Part model, mm, in its own coordinate system. A direction names the side the tool comes from. Round coordinates to 2 decimals unless told otherwise and drop trailing zeros. Loops run counter-clockwise (first coordinate to the right, second up) from the corner with the lowest first, then second, coordinate; pieces in that order, holes last.
1) Band-saw the part on C-C, the plane y = 65. Write the cut outline in (x, z).
2) Mould opens along Y. For faces 3 (the cylindrical face through (5.07, 55.357, -56.748)), 4 (the cylindrical face through (90.297, 5.07, -26.743)), 5 (the flat face through (115.07, 46.638, -102.915)) say: +Y half, -Y half, draft (parallel to the pull), parting line (faces both ways), or undercut.
3) Probe line 1 (X direction, y = 4.5, z = -20); line 2 (Z direction, x = 89.5, y = 9.5); line 3 (Y direction, x = 117, z = -60). List the from-to ranges inside material, lowest first.
4) Band-saw the part on B-B, the plane z = -20. Write the cut outline in (x, y).
5) Band-saw the part on D-D, the plane y = 52.5. Write the cut outline in (x, z), then the cut area to 3 significant figures.
6) 3-axis set-ups, long thin cutter, end or side, ignore diameter. For faces 1 (the flat face through (59, 10, -59)), 2 (the cylindrical face through (87.415, 5.07, -93.765)): which of +Z, -Z, +X, -X, +Y, -Y reach the whole face in a straight line?
7) Drop flat-ended pins along their axis: P1, Ø17.5, axis at x = 90, z = -20, coming from the +Y side; P2, Ø1.5, axis at x = 62.5, z = -72, coming from the -Y side. Give the stop position or say it passes through.
8) Band-saw the part on A-A, the plane x = 30. Write the cut outline in (y, z).
from build123d import *

# Parameters (mm, degrees)
ESQUISSE1_W             = 120
ESQUISSE1_H             = 120
BOSS_EXTRU_2_DEPTH      = 10
ESQUISSE2_R             = 15
BOSS_EXTRU_3_DEPTH      = 120
ESQUISSE3_W             = 100
ESQUISSE3_H             = 122.401822982
ENL_V_MAT_EXTRU_1_DEPTH = 197.482141726
ESQUISSE4_R             = 6.75
ENL_V_MAT_EXTRU_2_DEPTH = 10


with BuildPart() as part:
    # Esquisse1 → Boss.-Extru.2 (new body)
    with BuildSketch(Plane(origin=(0, 0, 0), x_dir=(1, 0, 0), z_dir=(0, 1, 0))):
        with Locations((60, 60)):
            Rectangle(ESQUISSE1_W, ESQUISSE1_H)
    extrude(amount=BOSS_EXTRU_2_DEPTH)

    # Esquisse2 → Boss.-Extru.3 (add)
    with BuildSketch(Plane(origin=(120, 0, 0), x_dir=(0, 0, -1), z_dir=(1, 0, 0))):
        with BuildLine():
            Line((86.302294997, 82.264961584), (120, 10))
            Line((120, 10), (0, 10))
            Line((0, 10), (33.697705003, 82.264961584))
            ThreePointArc((33.697705003, 82.264961584), (60, 99.021371518), (86.302294997, 82.264961584))
        make_face()
        with Locations((60, 70)):
            Circle(ESQUISSE2_R, mode=Mode.SUBTRACT)
    extrude(amount=-BOSS_EXTRU_3_DEPTH)

    # Esquisse3 → Enlèv. mat.-Extru.1 (cut, through all)
    with BuildSketch(Plane.XY):
        with Locations((60, 71.200911491)):
            Rectangle(ESQUISSE3_W, ESQUISSE3_H)
    extrude(amount=-ENL_V_MAT_EXTRU_1_DEPTH, mode=Mode.SUBTRACT)

    # Esquisse4 → Enlèv. mat.-Extru.2 (cut)
    with BuildSketch(Plane(origin=(0, 10, 0), x_dir=(1, 0, 0), z_dir=(0, 1, 0))):
        with Locations(Location((30, 20, 0), (0, 0, 270))):
            Circle(ESQUISSE4_R)
        with Locations(Location((30, 100, 0), (0, 0, 270))):
            Circle(ESQUISSE4_R)
        with Locations(Location((90, 100, 0), (0, 0, 270))):
            Circle(ESQUISSE4_R)
        with Locations(Location((90, 20, 0), (0, 0, 270))):
            Circle(ESQUISSE4_R)
    extrude(amount=-ENL_V_MAT_EXTRU_2_DEPTH, mode=Mode.SUBTRACT)


solid = part.part
Reported:
1. outline: (0, -94.35) - (10, -94.35) - (10, -74.14) - (0, -74.14) - close; (0, -45.86) - (10, -45.86) - (10, -25.65) - (0, -25.65) - close; (110, -94.35) - (120, -94.35) - (120, -74.14) - (110, -74.14) - close; (110, -45.86) - (120, -45.86) - (120, -25.65) - (110, -25.65) - close
2. face 3: undercut
2. face 4: draft
2. face 5: +Y half
3. line 1: x = 0 to 23.25, 36.75 to 83.25, 96.75 to 120
3. line 2: z = -120 to -106.73, -93.27 to -26.73, -13.27 to 0
3. line 3: y = 0 to 55, 85 to 99.02
4. outline: (0, 0) - (23.25, 0) - (23.25, 10) - (10, 10) - (10, 52.89) - (0, 52.89) - close; (36.75, 0) - (83.25, 0) - (83.25, 10) - (36.75, 10) - close; (96.75, 0) - (120, 0) - (120, 52.89) - (110, 52.89) - (110, 10) - (96.75, 10) - close
5. outline: (0, -100.18) - (10, -100.18) - (10, -19.82) - (0, -19.82) - close; (110, -100.18) - (120, -100.18) - (120, -19.82) - (110, -19.82) - close
5. area: 1,610 mm2
6. face 1: +Z, -Z, +Y
6. face 2: +Y, -Y
7. P1: stops at y = 10
7. P2: stops at y = 0
8. outline: (0, -120) - (10, -120) - (10, -106.75) - (0, -106.75) - close; (0, -93.25) - (10, -93.25) - (10, -26.75) - (0, -26.75) - close; (0, -13.25) - (10, -13.25) - (10, 0) - (0, 0) - close
